Geometry check sheet. Reference: the model listing, model coordinates, mm. A direction names the side the tool comes from. Coordinates: 2 decimals unless noted, no trailing zeros. Write each loop counter-clockwise with the first axis right and the second up, starting at its lowest first coordinate (ties: lowest second). Pieces come first, ordered by that corner, then holes. Notation, with made-up numbers: M -35.5,37.25 L -17.5,37.25 A20 cw -17.5,72.25 Z; hole C 49.25,13.25 d11. An arc over 180 degrees is marked long. Write each question's results on one line, items separated by ' | '.
```python
from build123d import *

# Parameters (mm, degrees)
SKETCH1_R           = 2.55
SKETCH1_R_2         = 2.5
SKETCH1_R_3         = 10
BOSS_EXTRUDE1_DEPTH = 6.35


with BuildPart() as part:
    # Sketch1 → Boss-Extrude1 (new body)
    with BuildSketch(Plane(origin=(0, 0, 0), x_dir=(1, 0, 0), z_dir=(0, 1, 0))):
        with BuildLine():
            Line((0, 42.5), (-147, 42.5))
            ThreePointArc((-147, 42.5), (-189.5, 0), (-147, -42.5))
            Line((-147, -42.5), (0, -42.5))
            ThreePointArc((0, -42.5), (42.5, 0), (0, 42.5))
        make_face()
        with BuildLine():
            Line((-147, 27.55), (-137, 27.55))
            ThreePointArc((-137, 27.55), (-134.45, 25), (-137, 22.45))
            Line((-137, 22.45), (-147, 22.45))
            ThreePointArc((-147, 22.45), (-149.55, 25), (-147, 27.55))
        make_face(mode=Mode.SUBTRACT)
        with Locations(Location((-147, 37.5, 0), (0, 0, 270))):
            Circle(SKETCH1_R, mode=Mode.SUBTRACT)
        with Locations(Location((-147, -37.5, 0), (0, 0, 270))):
            Circle(SKETCH1_R, mode=Mode.SUBTRACT)
        with BuildLine():
            ThreePointArc((-147, -27.55), (-149.55, -25), (-147, -22.45))
            Line((-147, -22.45), (-137, -22.45))
            ThreePointArc((-137, -22.45), (-134.45, -25), (-137, -27.55))
            Line((-137, -27.55), (-147, -27.55))
        make_face(mode=Mode.SUBTRACT)
        with Locations(Location((-184.5, 0, 0), (0, 0, 270))):
            Circle(SKETCH1_R, mode=Mode.SUBTRACT)
        with BuildLine():
            ThreePointArc((-172, -2.55), (-174.55, 0), (-172, 2.55))
            Line((-172, 2.55), (-162, 2.55))
            ThreePointArc((-162, 2.55), (-159.45, 0), (-162, -2.55))
            Line((-162, -2.55), (-172, -2.55))
        make_face(mode=Mode.SUBTRACT)
        with BuildLine():
            ThreePointArc((-147, -10), (-157, 0), (-147, 10))
            Line((-147, 10), (-137, 10))
            ThreePointArc((-137, 10), (-127, 0), (-137, -10))
            Line((-137, -10), (-147, -10))
        make_face(mode=Mode.SUBTRACT)
        with BuildLine():
            ThreePointArc((-122, -2.55), (-124.55, 0), (-122, 2.55))
            Line((-122, 2.55), (-112, 2.55))
            ThreePointArc((-112, 2.55), (-109.45, 0), (-112, -2.55))
            Line((-112, -2.55), (-122, -2.55))
        make_face(mode=Mode.SUBTRACT)
        with Locations(Location((0, 37.5, 0), (0, 0, 270))):
            Circle(SKETCH1_R, mode=Mode.SUBTRACT)
        with Locations(Location((0, -37.5, 0), (0, 0, 270))):
            Circle(SKETCH1_R, mode=Mode.SUBTRACT)
        with Locations(Location((-17.67766953, -17.67766953, 0), (0, 0, 270))):
            Circle(SKETCH1_R_2, mode=Mode.SUBTRACT)
        with Locations(Location((17.67766953, -17.67766953, 0), (0, 0, 270))):
            Circle(SKETCH1_R_2, mode=Mode.SUBTRACT)
        with Locations(Location((-17.67766953, 17.67766953, 0), (0, 0, 270))):
            Circle(SKETCH1_R_2, mode=Mode.SUBTRACT)
        with Locations(Location((0, 0, 0), (0, 0, 270))):
            Circle(SKETCH1_R_3, mode=Mode.SUBTRACT)
        with Locations(Location((37.5, 0, 0), (0, 0, 270))):
            Circle(SKETCH1_R, mode=Mode.SUBTRACT)
        with Locations(Location((17.67766953, 17.67766953, 0), (0, 0, 270))):
            Circle(SKETCH1_R_2, mode=Mode.SUBTRACT)
    extrude(amount=-BOSS_EXTRUDE1_DEPTH)


solid = part.part
```
Q1. Depth check by flat-ended pin: P1, Ø3, axis at x = -166, y = -3.5, coming from the +Z side; P2, Ø1, axis at y = -1.5, z = -10, coming from the +X side; P3, Ø1.5, axis at y = -1.5, z = -21.5, coming from the -X side. Enter the tip coordinate at first touch or a pass-through.
Geometry check:
P1: stops at z = 38.73 | P2: stops at x = 41.42 | P3: stops at x = -184.09
Q2. Access from +Z, -Z, +X, -X, +Y, -Y to the whole of each face (thin tool, end or side, straight path). Record for faces 4 (the cylindrical face through (-134.45, -3.13, 24.94)), 5 (the flat face through (-75, -3, 42.5)).
Geometry check:
face 4: +Y, -Y | face 5: +Z, +X, -X, +Y, -Y
Q3. Scan lines: probe 1 along X at (y, z) = (-1.25, 7); probe 2 along X at (y, z) = (-1.25, 18); probe 3 along X at (y, z) = (-4.75, 33). Record each from-to range of solid material in increasing order.
Geometry check:
probe 1: x = -188.92 to -154.14, -129.86 to -7.14, 7.14 to 41.92 | probe 2: x = -185.5 to -20.16, -15.2 to 15.2, 20.16 to 38.5 | probe 3: x = -173.78 to 26.78
Q4. Sectioned sample at C-C on x = -140. Record the cut outline in (y, z).
Geometry check:
outline: M -6.35,-42.5 L 0,-42.5 L 0,-27.55 L -6.35,-27.55 Z; M -6.35,-22.45 L 0,-22.45 L 0,-10 L -6.35,-10 Z; M -6.35,10 L 0,10 L 0,22.45 L -6.35,22.45 Z; M -6.35,27.55 L 0,27.55 L 0,42.5 L -6.35,42.5 Z
Q5. Sectioned sample at D-D on z = 25. Record the cut outline in (x, y), and give its area (3 significant figures).
Geometry check:
outline: M -181.37,-6.35 L -149.55,-6.35 L -149.55,0 L -181.37,0 Z; M -134.45,-6.35 L 34.37,-6.35 L 34.37,0 L -134.45,0 Z | area: 1,270 mm2
Q6. Sectioned sample at B-B on z = -37.5. Record the cut outline in (x, y), and give its area (3 significant figures).
Geometry check:
outline: M -167,-6.35 L -149.55,-6.35 L -149.55,0 L -167,0 Z; M -144.45,-6.35 L -2.55,-6.35 L -2.55,0 L -144.45,0 Z; M 2.55,-6.35 L 20,-6.35 L 20,0 L 2.55,0 Z | area: 1,120 mm2
Q7. Sectioned sample at A-A on x = 37.5. Record the cut outline in (y, z).
Geometry check:
outline: M -6.35,-20 L 0,-20 L 0,-2.55 L -6.35,-2.55 Z; M -6.35,2.55 L 0,2.55 L 0,20 L -6.35,20 Z
Q8. Mould release check, pull along X, two halves, no side actions. Record for faces 1 (the cylindrical face through (-174.55, -3.13, 0.06)), 2 (the flat face through (-75, -6.35, -1)), 3 (the cylindrical face through (42.49, -3.13, 0.93)): pulls with the +X half, pulls with the -X half, needs draft (parallel to the pull), parting line crosses it, or undercut.
Geometry check:
face 1: undercut | face 2: needs draft | face 3: pulls with the +X half
